Part model, mm, in its own coordinate system. A direction names the side the tool comes from. Give positions to 0.01 mm unless a question says otherwise; leave off trailing zeros. Order: outer loops, then holes, each group sorted by start corner. A loop starts at its lowest first (then second) coordinate and runs counter-clockwise, first axis right, second up. Notation, with made-up numbers: (73, 14) - (112, 14) arc R36 ccw to (112, 48) - close; hole circle Ø1 at (-8, 4.5). An arc over 180 degrees is marked (long way). One line per item, written item: value.
```python
from build123d import *

# Parameters (mm, degrees)
SKETCH1_R           = 2.38125
SKETCH1_R_2         = 20.955
BOSS_EXTRUDE1_DEPTH = 4.7625
SKETCH2_R           = 2.38125
CUT_EXTRUDE1_DEPTH  = 343.797654481
FILLET1_R           = 38.1
SKETCH4_R           = 2.38125
CUT_EXTRUDE3_DEPTH  = 343.797654481
FILLET2_R           = 38.1
CUT_EXTRUDE4_DEPTH  = 338.871506933
FILLET3_R           = 12.7


with BuildPart() as part:
    # Sketch1 → Boss-Extrude1 (new body)
    with BuildSketch(Plane(origin=(0, 0, 0), x_dir=(1, 0, 0), z_dir=(0, 1, 0))):
        with BuildLine():
            Line((63.5, 31.75), (63.5, 292.608))
            Line((63.5, 292.608), (-63.5, 292.608))
            Line((-63.5, 292.608), (-63.5, 31.75))
            Line((-63.5, 31.75), (-178.516410583, -97.067662754))
            ThreePointArc((-178.516410583, -97.067662754), (-152.483723292, -134.309173667), (-118.826410583, -164.834838999))
            Line((-118.826410583, -164.834838999), (0, -31.75))
            Line((0, -31.75), (118.826410583, -164.834838999))
            ThreePointArc((118.826410583, -164.834838999), (152.483723292, -134.309173667), (178.516410583, -97.067662754))
            Line((178.516410583, -97.067662754), (63.5, 31.75))
        make_face()
        with Locations(Location((-25.4, 0, 0), (0, 0, 90))):
            Circle(SKETCH1_R, mode=Mode.SUBTRACT)
        with Locations(Location((0, 0, 0), (0, 0, 90))):
            Circle(SKETCH1_R_2, mode=Mode.SUBTRACT)
        with Locations(Location((25.4, 0, 0), (0, 0, 90))):
            Circle(SKETCH1_R, mode=Mode.SUBTRACT)
    extrude(amount=BOSS_EXTRUDE1_DEPTH)

    # Sketch2 → Cut-Extrude1 (cut, through all)
    with BuildSketch(Plane(origin=(0, 4.7625, 0), x_dir=(1, 0, 0), z_dir=(0, 1, 0))):
        with Locations(Location((25.4, 279.908, 0), (0, 0, 270))):
            Circle(SKETCH2_R)
        with Locations(Location((50.8, 279.908, 0), (0, 0, 270))):
            Circle(SKETCH2_R)
        with Locations(Location((-50.8, 279.908, 0), (0, 0, 270))):
            Circle(SKETCH2_R)
        with Locations(Location((-25.4, 279.908, 0), (0, 0, 270))):
            Circle(SKETCH2_R)
    extrude(amount=-CUT_EXTRUDE1_DEPTH, mode=Mode.SUBTRACT)

    # Fillet1
    fillet1_edges = [part.edges().sort_by_distance(p)[0] for p in [
        (63.5, 2.38125, -31.75),
        (0, 2.38125, 31.75),
        (-63.5, 2.38125, -31.75),
    ]]
    fillet(fillet1_edges, radius=FILLET1_R)

    # Sketch4 → Cut-Extrude3 (cut, through all)
    with BuildSketch(Plane(origin=(0, 4.7625, 0), x_dir=(1, 0, 0), z_dir=(0, 1, 0))):
        with Locations(Location((-156.048464437, -109.266311125, 0), (0, 0, 270))):
            Circle(SKETCH4_R)
        with Locations(Location((-126.479111192, -142.454499515, 0), (0, 0, 270))):
            Circle(SKETCH4_R)
        with Locations(Location((126.479111192, -142.454499515, 0), (0, 0, 270))):
            Circle(SKETCH4_R)
        with Locations(Location((156.048464437, -109.266311125, 0), (0, 0, 270))):
            Circle(SKETCH4_R)
    extrude(amount=-CUT_EXTRUDE3_DEPTH, mode=Mode.SUBTRACT)

    # Fillet2
    fillet2_edges = [part.edges().sort_by_distance(p)[0] for p in [
        (178.516410583, 2.38125, 97.067662754),
        (-178.516410583, 2.38125, 97.067662754),
    ]]
    fillet(fillet2_edges, radius=FILLET2_R)

    # Sketch5 → Cut-Extrude4 (cut, through all)
    with BuildSketch(Plane(origin=(0, 4.7625, 0), x_dir=(1, 0, 0), z_dir=(0, 1, 0))):
        Polygon((-149.276482194, -103.59593683), (-111.382942554, -137.429642709), (-69.090810204, -90.062718159), (-106.984349844, -56.22901228), align=None)
        Polygon((106.984349844, -56.22901228), (69.090810204, -90.062718159), (111.382942554, -137.429642709), (149.276482194, -103.59593683), align=None)
    extrude(amount=-CUT_EXTRUDE4_DEPTH, mode=Mode.SUBTRACT)

    # Fillet3
    fillet3_edges = [part.edges().sort_by_distance(p)[0] for p in [
        (-149.276482194, 2.38125, 103.59593683),
        (-106.984349844, 2.38125, 56.22901228),
        (-69.090810204, 2.38125, 90.062718159),
        (-111.382942554, 2.38125, 137.429642709),
        (106.984349844, 2.38125, 56.22901228),
        (149.276482194, 2.38125, 103.59593683),
        (111.382942554, 2.38125, 137.429642709),
        (69.090810204, 2.38125, 90.062718159),
    ]]
    fillet(fillet3_edges, radius=FILLET3_R)


solid = part.part
```
1) Slice it at C-C on y = 3.6. Count the separate pieces of the cut face and the enclosed holes in it, then the cut area to 3 significant figures.
Answer:
separate pieces: 1
enclosed holes: 13
area: 61,600 mm2
2) Slice it at A-A on x = 0. Write the cut outline in (y, z) (1 decimal).
Answer:
outline: (0, -292.6) - (4.8, -292.6) - (4.8, -21) - (0, -21) - close; (0, 21) - (4.8, 21) - (4.8, 50.9) - (0, 50.9) - close
3) Wall check: line 1 along X through (y, z) = (3.25, 85.5); line 2 along X through (y, z) = (3.8, 126); line 3 along Z through (x, y) = (127, 0.65). Give the ranges that are in metal, low to high. Write a range as [from, to].
Answer:
line 1: x = [-165.66, -133.12], [-75.61, -47.99], [47.99, 75.61], [133.12, 165.66]
line 2: x = [-159.42, -124.18], [-101.18, -84.15], [84.15, 101.18], [124.18, 159.42]
line 3: z = [39.37, 78.65], [123.49, 140.13], [144.78, 158.62]
4) Two-plate mould, pull along Z, no slides. Class faces 1 (the face through (-130.462, 2.415, 120.394)), 2 (the face through (-168.824, 2.415, 99.047)), 3 (the face through (-87.905, 2.415, 73.264)), 4 (the face through (-74.26, 2.35, 114.92)): pulls with the +Z half, pulls with the -Z half, needs draft (parallel to the pull), parting line crosses it, or undercut.
Answer:
face 1: undercut
face 2: parting line crosses it
face 3: undercut
face 4: pulls with the +Z half
5) Slice it at D-D on x = -86.5. Write the cut outline in (y, z).
Answer:
outline: (0, -5.99) - (4.76, -5.99) - (4.76, 74.52) - (0, 74.52) - close; (0, 109.56) - (4.76, 109.56) - (4.76, 128.63) - (0, 128.63) - close
6) Slice it at B-B on z = -231. Write the cut outline in (x, y), then the cut area to 3 significant figures.
Answer:
outline: (-63.5, 0) - (63.5, 0) - (63.5, 4.76) - (-63.5, 4.76) - close
area: 605 mm2
7) Which spindle directions (+Z, -Z, +X, -X, +Y, -Y) get a long thin tool onto all of the face, cutting with end or side? Do faces 5 (the face through (72.99, 2.35, 113.5)), 6 (the face through (116.784, 2.348, 27.928)), 7 (the face through (-90.415, 2.415, 113.945)). Say none if no direction does.
Answer:
face 5: +Z, +Y, -Y
face 6: -Z, +X, +Y, -Y
face 7: +Y, -Y
8) Drop flat-ended pins along their axis: P1, Ø5.5, axis at x = 156.05, z = 109.27, coming from the +Y side; P2, Ø2.5, axis at y = 3, z = -119.5, coming from the -X side; P3, Ø2, axis at y = 2, z = 64.5, coming from the +X side; P4, Ø1, axis at x = 34.5, y = 4, coming from the +Z side. Give the stop position or say it passes through.
Answer:
P1: stops at y = 4.76
P2: stops at x = -63.5
P3: stops at x = 150.33
P4: stops at z = 70.95
